```python
from build123d import *

# Parameters (mm, degrees)
SKETCH_1_W      = 120
SKETCH_1_H      = 70
EXTRUDE_1_DEPTH = 5
SKETCH_2_W      = 120
SKETCH_2_H      = 70
EXTRUDE_2_DEPTH = 5
SKETCH_3_W      = 8
SKETCH_3_H      = 72
SKETCH_3_W_2    = 72
SKETCH_3_H_2    = 8
EXTRUDE_3_DEPTH = 50
SKETCH_4_W      = 300
SKETCH_4_H      = 300
EXTRUDE_4_DEPTH = 5
EXTRUDE_5_DEPTH = 5


with BuildPart() as part:
    # 草图1 → 凸台-拉伸1 (new body)
    with BuildSketch(Plane(origin=(0, 0, 0), x_dir=(1, 0, 0), z_dir=(0, 1, 0))):
        Polygon((-150, 150), (150, 150), (150, -30), (150, -150), (0, -150), (-150, -150), align=None)
        Polygon((-15.857864376, 30), (120, 30), (120, -30), (44.142135624, -30), align=None, mode=Mode.SUBTRACT)
        Polygon((-105.857864376, 120), (120, 120), (120, 50), (-35.857864376, 50), align=None, mode=Mode.SUBTRACT)
        Polygon((-120, 105.857864376), (-120, 50), (-64.142135624, 50), align=None, mode=Mode.SUBTRACT)
        with Locations((-60, -85)):
            Rectangle(SKETCH_1_W, SKETCH_1_H, mode=Mode.SUBTRACT)
        Polygon((-120, 30), (-44.142135624, 30), (15.857864376, -30), (-120, -30), align=None, mode=Mode.SUBTRACT)
    extrude(amount=EXTRUDE_1_DEPTH)

    # 草图2 → 凸台-拉伸2 (add)
    with BuildSketch(Plane.XZ):
        with BuildLine():
            Line((150, 45), (150, 150))
            Line((150, 150), (-150, 150))
            Line((-150, 150), (-150, -150))
            Line((-150, -150), (150, -150))
            Line((150, -150), (150, -45))
            Line((150, -45), (-110, -45))
            ThreePointArc((-110, -45), (-111.913417162, -44.619397663), (-113.535533906, -43.535533906))
            ThreePointArc((-113.535533906, -43.535533906), (-115, -42.928932188), (-116.464466094, -43.535533906))
            ThreePointArc((-116.464466094, -43.535533906), (-125, -40), (-116.464466094, -36.464466094))
            ThreePointArc((-116.464466094, -36.464466094), (-115, -37.071067812), (-113.535533906, -36.464466094))
            ThreePointArc((-113.535533906, -36.464466094), (-111.913417162, -35.380602337), (-110, -35))
            Line((-110, -35), (150, -35))
            Line((150, -35), (150, 35))
            Line((150, 35), (-110, 35))
            ThreePointArc((-110, 35), (-111.913417162, 35.380602337), (-113.535533906, 36.464466094))
            ThreePointArc((-113.535533906, 36.464466094), (-115, 37.071067812), (-116.464466094, 36.464466094))
            ThreePointArc((-116.464466094, 36.464466094), (-125, 40), (-116.464466094, 43.535533906))
            ThreePointArc((-116.464466094, 43.535533906), (-115, 42.928932188), (-113.535533906, 43.535533906))
            ThreePointArc((-113.535533906, 43.535533906), (-111.913417162, 44.619397663), (-110, 45))
            Line((-110, 45), (150, 45))
        make_face()
        with Locations((-60, 85)):
            Rectangle(SKETCH_2_W, SKETCH_2_H, mode=Mode.SUBTRACT)
        Polygon((-120, 30), (-120, -30), (-44.142135624, -30), (15.857864376, 30), align=None, mode=Mode.SUBTRACT)
        Polygon((44.142135624, 30), (-15.857864376, -30), (120, -30), (120, 30), align=None, mode=Mode.SUBTRACT)
        Polygon((-120, -50), (-120, -105.857864376), (-64.142135624, -50), align=None, mode=Mode.SUBTRACT)
        Polygon((-35.857864376, -50), (-105.857864376, -120), (120, -120), (120, -50), align=None, mode=Mode.SUBTRACT)
    extrude(amount=EXTRUDE_2_DEPTH)

    # 草图3 → 凸台-拉伸3 (add)
    with BuildSketch(Plane(origin=(0, 5, 0), x_dir=(1, 0, 0), z_dir=(0, 1, 0))):
        with Locations((146, -106)):
            Rectangle(SKETCH_3_W, SKETCH_3_H)
        with Locations((-106, -146)):
            Rectangle(SKETCH_3_W_2, SKETCH_3_H_2)
        with Locations((-146, 106)):
            Rectangle(SKETCH_3_W, SKETCH_3_H)
        with Locations((106, 146)):
            Rectangle(SKETCH_3_W_2, SKETCH_3_H_2)
    extrude(amount=EXTRUDE_3_DEPTH)

    # 草图4 → 凸台-拉伸4 (add)
    with BuildSketch(Plane(origin=(0, 55, 0), x_dir=(1, 0, 0), z_dir=(0, 1, 0))):
        Rectangle(SKETCH_4_W, SKETCH_4_H)
        Polygon((30, 120), (-30, 120), (-30, -15.857864376), (30, 44.142135624), align=None, mode=Mode.SUBTRACT)
        Polygon((105.857864376, 120), (50, 120), (50, 64.142135624), align=None, mode=Mode.SUBTRACT)
        Polygon((120, 105.857864376), (120, -120), (50, -120), (50, 35.857864376), align=None, mode=Mode.SUBTRACT)
        Polygon((-120, 120), (-120, -105.857864376), (-50, -35.857864376), (-50, 120), align=None, mode=Mode.SUBTRACT)
        Polygon((-50, -120), (-105.857864376, -120), (-50, -64.142135624), align=None, mode=Mode.SUBTRACT)
        Polygon((30, -120), (-30, -120), (-30, -44.142135624), (30, 15.857864376), align=None, mode=Mode.SUBTRACT)
    extrude(amount=EXTRUDE_4_DEPTH)

    # 草图5 → 凸台-拉伸5 (add)
    with BuildSketch(Plane(origin=(0, 60, 0), x_dir=(1, 0, 0), z_dir=(0, 1, 0))):
        with BuildLine():
            Line((35, 110), (35, -150))
            Line((35, -150), (45, -150))
            Line((45, -150), (45, 110))
            ThreePointArc((45, 110), (44.619397663, 111.913417162), (43.535533906, 113.535533906))
            ThreePointArc((43.535533906, 113.535533906), (42.928932188, 115), (43.535533906, 116.464466094))
            ThreePointArc((43.535533906, 116.464466094), (40, 125), (36.464466094, 116.464466094))
            ThreePointArc((36.464466094, 116.464466094), (37.071067812, 115), (36.464466094, 113.535533906))
            ThreePointArc((36.464466094, 113.535533906), (35.380602337, 111.913417162), (35, 110))
        make_face()
        with BuildLine():
            Line((-45, -150), (-35, -150))
            Line((-35, -150), (-35, 110))
            ThreePointArc((-35, 110), (-35.380602337, 111.913417162), (-36.464466094, 113.535533906))
            ThreePointArc((-36.464466094, 113.535533906), (-37.071067812, 115), (-36.464466094, 116.464466094))
            ThreePointArc((-36.464466094, 116.464466094), (-40, 125), (-43.535533906, 116.464466094))
            ThreePointArc((-43.535533906, 116.464466094), (-42.928932188, 115), (-43.535533906, 113.535533906))
            ThreePointArc((-43.535533906, 113.535533906), (-44.619397663, 111.913417162), (-45, 110))
            Line((-45, 110), (-45, -150))
        make_face()
    extrude(amount=EXTRUDE_5_DEPTH)


solid = part.part
```
The listing builds one solid part. Answer for the finished solid, in the listing's coordinates (mm). A direction names the side the tool comes from. Give positions to 0.01 mm unless a question says otherwise; leave off trailing zeros. Order: outer loops, then holes, each group sorted by start corner. A loop starts at its lowest first (then second) coordinate and runs counter-clockwise, first axis right, second up. Notation, with made-up numbers: (-22.75, 66) -> (1.25, 66) arc R24 ccw to (1.25, 80) -> close; hole circle Ø11 at (29, -17.5). An arc over 180 degrees is marked (long way). One line per item, written item: value.
1) A tool of negligible diameter and unlimited length cuts with its end or side. For faces 1 (the flat face through (120, 0, 0)), 2 (the flat face through (-2, 55, -2)), 3 (the flat face through (-146, 30, -142)), from which of +Z, -Z, +X, -X, +Y, -Y can it reach the whole face along a straight path? Write none if from no direction.
Reported:
face 1: +Y, -Y
face 2: none
face 3: -Z, -X
2) Flat-ended cylindrical pins translate along their axes: P1, Ø4, axis at x = 75.5, z = 30.5, coming from the +Y side; P2, Ø9, axis at x = -146, y = 36, coming from the -Z side; P3, Ø6.5, axis at y = 22.5, z = 147.5, coming from the -X side. Find the tip coordinate at first contact, or state that the pin passes through.
Reported:
P1: stops at y = 5
P2: stops at z = -142
P3: stops at x = -142
3) Determine the mould class of faces 4 (the flat face through (65, 56, -150)), 5 (the flat face through (-0.42, 57.46, -13.72)), 6 (the flat face through (84.51, 57.46, -70.37)), 7 (the flat face through (70, 30, -146)) for opening direction Z: pulls with the +Z half, pulls with the -Z half, needs draft (parallel to the pull), parting line crosses it, or undercut.
Reported:
face 4: pulls with the -Z half
face 5: undercut
face 6: undercut
face 7: needs draft
4) Find the intervals of material crossed by line 1 (X direction, y = 4.5, z = 65.5); line 2 (X direction, y = 3.5, z = -8); line 3 (Y direction, x = -125.5, z = -97.5), in increasing order.
Reported:
line 1: x = -150 to -120, 0 to 150
line 2: x = -150 to -120, -22.14 to 6.14, 120 to 150
line 3: y = -5 to 5, 55 to 60
5) Find section A-A, the plane y = 26.5. Determine the outline of the cut face in (x, z).
Reported:
outline: (-150, -142) -> (-142, -142) -> (-142, -70) -> (-150, -70) -> close; (-142, 142) -> (-70, 142) -> (-70, 150) -> (-142, 150) -> close; (70, -150) -> (142, -150) -> (142, -142) -> (70, -142) -> close; (142, 70) -> (150, 70) -> (150, 142) -> (142, 142) -> close
6) Find section B-B, the plane x = 55. Count the separate pieces of the cut face and the enclosed holes in it, plus the area to 3 significant figures.
Reported:
separate pieces: 6
enclosed holes: 0
area: 2,040 mm^2
